Build history of the part. All positions in model axes, mm. A direction names the side the tool comes from. Round coordinates to 2 decimals unless told otherwise and drop trailing zeros. Order: outer loops, then holes, each group sorted by start corner. A loop starts at its lowest first (then second) coordinate and runs counter-clockwise, first axis right, second up. Notation, with made-up numbers: (34.5, 42.5) -> (74.5, 42.5) arc R20 ccw to (74.5, 57.5) -> close; hole circle Ø4 at (85.5, 8). An arc over 180 degrees is marked (long way). Use a Markdown table: item, result. Add a question column.
Item 1: Slice it at D-D, the plane y = -59.5. Give the cut face in (x, z), plus the area to 3 significant figures.
Item 2: Slice it at B-B, the plane z = 15. Give the cut face in (x, y) (3 decimals), plus the area to 3 significant figures.
Item 3: Slice it at C-C, the plane x = -96. Give the cut face in (y, z), plus the area to 3 significant figures.
Item 4: 3-axis set-ups, long thin cutter, end or side, ignore diameter. For faces 1 (the face through (-2, -26, 6.35)), 2 (the face through (52.084, -78.523, 3.131)): which of +Z, -Z, +X, -X, +Y, -Y reach the whole face in a straight line?
Item 5: Slice it at A-A, the plane y = 0. Give the cut face in (x, z) (3 decimals).
Item 6: Two-plate mould, pull along X, no slides. Class faces 3 (the face through (11.746, 15.319, 3.131)), 4 (the face through (-103.3, 79.21, 28.17)), 5 (the face through (87.9, 21.78, 3.13)), 6 (the face through (48, -115, 57.15)): released by +X, released by -X, zero draft, split by the parting line, or undercut.
Item 7: Pin check, flat tips, straight feed: pin 1 (3 mm diameter, centred on y = 125.5, z = 59, fed in from +X); pin 2 (8 mm diameter, centred on x = -84.55, y = 27.47, fed in from +Z); pin 3 (12 mm diameter, centred on x = -72, z = 25, fed in from +Y); pin 4 (1.5 mm diameter, centred on x = 20, z = 7, fed in from +Y). Stop position of each tip, or through.
Item 8: Probe L1, parallel to Y at x = 1, z = 26; L2, parallel to Z at x = -105, y = -0.5; L3, parallel to Y at x = 86.5, z = 55. List the from-to ranges inside material, lowest first.
Autodesk Inventor part; units mm, degrees
ref_plane "YZ Plane" through (0, 0, 0) normal (1, 0, 0) x (0, 1, 0)
ref_plane "XZ Plane" through (0, 0, 0) normal (0, 1, 0) x (-1, 0, 0)
ref_plane "XY Plane" through (0, 0, 0) normal (0, 0, 1) x (1, 0, 0)
sketch "Sketch1" plane through (0, 0, 0) normal (0, 0, 1) x (1, 0, 0)
  circle A0 centre (0, 0) radius 130.175
  dimension "d0" = 260.35
extrude "Extrusion1" add sketch "Sketch1" along normal blind 6.35
sketch "Sketch2" plane through (0, 0, 6.35) normal (0, 0, 1) x (1, 0, 0)
  circle A0 centre (0, 0) radius 130.175
  circle A1 centre (0, 0) radius 123.825
  dimension "d3" = 6.35
extrude "Extrusion2" add sketch "Sketch2" along normal blind 50.8
sketch "Sketch4" plane through (0, 0, 6.35) normal (0, 0, 1) x (1, 0, 0)
  point P0 (0, 0)
  point P1 (0, 0)
hole "Hole1" at (0, 0, 6.35) direction (0, 0, -1) diameter 38.608 end through all
sketch "Sketch5" plane through (0, 0, 6.35) normal (0, 0, 1) x (1, 0, 0)
  point P0 (0, 0)
  point P1 (0, 88.9)
  dimension "d13" = 88.9
hole "Hole2" at (0, 88.9, 6.35) direction (0, 0, -1) diameter 13.208 end through all
pattern_circular "Circular Pattern1" count 5 over 360 about axis through (0, 0, -366.2495) along (0, 0, 1) of "Hole2"
sketch "Sketch7" plane through (-0.7894, 85.7534, 57.15) normal (0, 0, 1) x (1, 0, 0)
  line L0 (-3.175, 44.45) -> (3.175, 44.45)
  line L1 (3.175, 44.45) -> (3.175, 38.1)
  line L2 (3.175, 38.1) -> (-3.175, 38.1)
  line L3 (-3.175, 38.1) -> (-3.175, 44.45)
  point P0 (0, 0)
  dimension "d35" = 6.35
  dimension "d36" = 6.35
  dimension "d33" = 3.175
  dimension "d34" = 44.45
extrude "Extrusion4" add sketch "Sketch7" along normal blind 6.35
fillet "Fillet1" radius 2.54 4 edges at (-0.7894, 130.2034, 63.5) (2.3856, 127.0284, 63.5) (-0.7894, 123.8534, 63.5) (-3.9644, 127.0284, 63.5)
equation "\"d0\" = W_innerDiameter + W_wallThickness"
equation "\"d1\" = W_wallThickness"
equation "\"d3\" = W_wallThickness"
equation "\"d4\" = W_innerDepth"
equation "\"d6\" = W_innerGearHoleDiameter"
equation "\"d14\" = W_outerGearHoleDiameter"
equation "\"d39\" = d41"
equation "\"W_wallThickness\" = 6.35"
equation "\"W_innerDepth\" = 50.8"
equation "\"W_innerGearHoleDiameter\" = 38.608"
equation "\"W_outerGearHoleDiameter\" = 13.208"
equation "\"OG_distanceFromCenter\" = 88.9"
equation "\"W_innerDiameter\" = 254"
equation "\"Wheel_Related_W_\" = 0"
equation "\"W_holesClearance\" = 0.254"
equation "\"TempSpotReserved7\" = 0"
equation "\"TempSpotReserved8\" = 0"
equation "\"TempSpotReserved9\" = 0"
equation "\"TempSpotReserved10\" = 0"
equation "\"TempSpotReserved11\" = 0"
equation "\"TempSpotReserved12\" = 0"
equation "\"TempSpotReserved13\" = 0"
equation "\"TempSpotReserved14\" = 0"
equation "\"TempSpotReserved15\" = 0"
equation "\"TempSpotReserved16\" = 0"
equation "\"TempSpotReserved17\" = 0"
equation "\"TempSpotReserved18\" = 0"
equation "\"TempSpotReserved19\" = 0"
equation "\"TempSpotReserved20\" = 0"
equation "\"Inner_Gear_Related_IG_\" = 0"
equation "\"IG_shaftDiameter\" = 25.4"
equation "\"IG_gearDiameter\" = 127"
equation "\"IG_shaftLength\" = 127"
equation "\"IG_gearThickness\" = 6.35"
equation "\"TempSpotReserved25\" = 0"
equation "\"TempSpotReserved26\" = 0"
equation "\"TempSpotReserved27\" = 0"
equation "\"TempSpotReserved28\" = 0"
equation "\"TempSpotReserved29\" = 0"
equation "\"TempSpotReserved30\" = 0"
equation "\"TempSpotReserved31\" = 0"
equation "\"TempSpotReserved32\" = 0"
equation "\"TempSpotReserved33\" = 0"
equation "\"TempSpotReserved34\" = 0"
equation "\"TempSpotReserved35\" = 0"
equation "\"TempSpotReserved36\" = 0"
equation "\"TempSpotReserved37\" = 0"
equation "\"TempSpotReserved38\" = 0"
equation "\"TempSpotReserved39\" = 0"
equation "\"TempSpotReserved40\" = 0"
equation "\"Outer_Gear_Related_OG_\" = 0"
equation "\"OG_shaftDiameter\" = 12.7"
equation "\"OG_gearDiameter\" = 50.8"
equation "\"OG_shaftLength\" = 57.15"
equation "\"OG_gearThickness\" = 6.35"
equation "\"TempSpotReserved47\" = 0"
equation "\"TempSpotReserved48\" = 0"
equation "\"TempSpotReserved49\" = 0"
equation "\"TempSpotReserved50\" = 0"
equation "\"TempSpotReserved51\" = 0"
equation "\"TempSpotReserved52\" = 0"
equation "\"TempSpotReserved53\" = 0"
equation "\"TempSpotReserved54\" = 0"
equation "\"TempSpotReserved55\" = 0"
equation "\"TempSpotReserved56\" = 0"
equation "\"TempSpotReserved57\" = 0"
equation "\"TempSpotReserved58\" = 0"
equation "\"TempSpotReserved59\" = 0"
equation "\"TempSpotReserved60\" = 0"
equation "\"Leg_Extensions_Related_LE_\" = 0"
equation "\"LE_baseDiameter\" = 19.05"
equation "\"LE_maxLength\" = 93.92488"
equation "\"LE_thickness\" = 19.05"
equation "\"IG_ratioToOuterGear\" = 2.5"
equation "\"B_bearingThickness\" = 6.35"
equation "\"TempSpotReserved43\" = 0"
equation "\"TempSpotReserved45\" = 0"
equation "\"Thisisatest\" = 25.4"
equation "\"TempSpotReserved46\" = 0"
equation "\"TempSpotReserved44\" = 0"
equation "\"LE_offsetAboveOuterGear\" = 0"
equation "\"Bearing_Related_B_\" = 0"
equation "\"TempSpotReserved42\" = 0"
properties part number "Wheel_1"
Check sheet entries:
| question | item | result |
|---|---|---|
| 1 | outline | (-115.78, 0) -> (115.78, 0) -> (115.78, 57.15) -> (108.59, 57.15) -> (108.59, 6.35) -> (-108.59, 6.35) -> (-108.59, 57.15) -> (-115.78, 57.15) -> close |
| 1 | area | 2,200 mm2 |
| 2 | outline | circle Ø260.35 at (0, 0); hole circle Ø247.65 at (0, 0) |
| 2 | area | 5,070 mm2 |
| 3 | outline | (-87.92, 0) -> (87.92, 0) -> (87.92, 57.15) -> (78.21, 57.15) -> (78.21, 6.35) -> (-78.21, 6.35) -> (-78.21, 57.15) -> (-87.92, 57.15) -> close |
| 3 | area | 2,100 mm2 |
| 4 | face 1 | +Z |
| 4 | face 2 | +Z, -Z |
| 5 | outline | (-130.175, 0) -> (-19.304, 0) -> (-19.304, 6.35) -> (-123.825, 6.35) -> (-123.825, 57.15) -> (-130.175, 57.15) -> close; (19.304, 0) -> (130.175, 0) -> (130.175, 57.15) -> (123.825, 57.15) -> (123.825, 6.35) -> (19.304, 6.35) -> close |
| 6 | face 3 | undercut |
| 6 | face 4 | split by the parting line |
| 6 | face 5 | undercut |
| 6 | face 6 | zero draft |
| 7 | pin 1 | x = 2.39 |
| 7 | pin 2 | through |
| 7 | pin 3 | y = 112.2 |
| 7 | pin 4 | y = 128.74 |
| 8 | L1 | -130.17 to -123.82, 123.82 to 130.17 |
| 8 | L2 | 0 to 6.35 |
| 8 | L3 | -97.28 to -88.6, 88.6 to 97.28 |
